Source: CAD feature listing. Evaluate the final solid. Frame: model axes, mm. A direction names the side the tool comes from. Give positions to 0.01 mm unless a question says otherwise; leave off trailing zeros. Order: outer loops, then holes, each group sorted by start corner. A loop starts at its lowest first (then second) coordinate and runs counter-clockwise, first axis right, second up. Notation, with made-up numbers: (64, 10.25) - (113, 10.25) arc R18 cw to (113, 30.25) - close; hole circle Ø4 at (-6.75, -8.75). An arc over 180 degrees is marked (long way). Use CSV: the item, a comma, the result in double quotes.
```python
from build123d import *

# Parameters (mm, degrees)
CROQUIS1_R              = 19
SALIENTE_EXTRUIR1_DEPTH = 50
CHAFL_N1_SIZE           = 2
CROQUIS2_R              = 8
CORTAR_EXTRUIR1_DEPTH   = 30


with BuildPart() as part:
    # Croquis1 → Saliente-Extruir1 (new body)
    with BuildSketch(Plane.XY):
        Circle(CROQUIS1_R)
    extrude(amount=-SALIENTE_EXTRUIR1_DEPTH)

    # Chaflán1
    chafl_n1_edges = [part.edges().sort_by_distance(p)[0] for p in [
        (-19, 0, 0),
    ]]
    chamfer(chafl_n1_edges, length=CHAFL_N1_SIZE)

    # Croquis2 → Cortar-Extruir1 (cut)
    with BuildSketch(Plane(origin=(0, 0, -50), x_dir=(-1, 0, 0), z_dir=(0, 0, -1))):
        Circle(CROQUIS2_R)
    extrude(amount=-CORTAR_EXTRUIR1_DEPTH, mode=Mode.SUBTRACT)


solid = part.part
```
Item 1: Mould query, pull axis X, two halves, no side actions, for faces 1 (the flat face through (0, 0, -20)), 2 (the cylindrical face through (8.767, -16.856, -25.664)), 3 (the flat face through (0, 0, 0)). Classes: released by +X, released by -X, zero draft, split by the parting line, or undercut.
Filled in:
face 1,"undercut"
face 2,"split by the parting line"
face 3,"zero draft"
Item 2: Section A-A on y = 0. Return the cut outline in (x, z).
Filled in:
outline,"(-19, -50) - (-8, -50) - (-8, -20) - (8, -20) - (8, -50) - (19, -50) - (19, -2) - (17, 0) - (-17, 0) - (-19, -2) - close"
Item 3: Set-up query: faces 4 (the flat face through (8.2, 0.3, -50)), 5 (the cylindrical face through (1.73, -7.81, -35.21)). Return all of +Z, -Z, +X, -X, +Y, -Y with unobstructed straight access to the full face (end or side cutting, diameter ignored); none if empty.
Filled in:
face 4,"-Z, +X, -X, +Y, -Y"
face 5,"-Z"
Item 4: Material intervals for line 1 (Y direction, x = 0, z = -35.25); line 2 (Y direction, x = 0.5, z = -13.5); line 3 (Z direction, x = 4.5, y = -4), sorted ascending. Write a range as from..to.
Filled in:
line 1,"y = -19..-8, 8..19"
line 2,"y = -18.99..18.99"
line 3,"z = -20..0"
Item 5: Section C-C on z = -10.5. Return the cut outline in (x, y), then the cut area to 3 significant figures.
Filled in:
outline,"circle Ø38 at (0, 0)"
area,"1,130 mm2"
Item 6: Section D-D on z = -30. Return the cut outline in (x, y).
Filled in:
outline,"circle Ø38 at (0, 0); hole circle Ø16 at (0, 0)"
Item 7: First-contact query: pin 1 (10 mm diameter, centred on x = 0.5, y = -2, fed in from -Z); pin 2 (1.5 mm diameter, centred on y = 2, z = -23, fed in from +X); pin 3 (1.5 mm diameter, centred on x = -6, z = -25, fed in from +Y). Flat tips, straight axial feed; report the tip coordinate or a pass-through.
Filled in:
pin 1,"stops at z = -20"
pin 2,"stops at x = 18.96"
pin 3,"stops at y = 18.26"
